The listing builds one solid part. Answer for the finished solid, in the listing's coordinates (mm). A direction names the side the tool comes from. Round coordinates to 2 decimals unless told otherwise and drop trailing zeros. Write each loop counter-clockwise with the first axis right and the second up, starting at its lowest first coordinate (ties: lowest second). Pieces come first, ordered by that corner, then holes. Notation, with made-up numbers: (-36.75, 71) - (-4.75, 71) arc R20 cw to (-4.75, 101) - close; hole circle Ø2 at (-13.75, 50.5). An arc over 180 degrees is marked (long way). Answer in a Markdown table with one row per item.
from build123d import *

# Parameters (mm, degrees)
F0_W     = 58
F0_H     = 63
F1_DEPTH = 29.5
F2_R     = 5
F3_R     = 4
F3_R_2   = 2.5
F4_DEPTH = 4


with BuildPart() as f1:
    # F0 (on Front) → F1 (new body)
    with BuildSketch(Plane.XZ):
        Rectangle(F0_W, F0_H)
    extrude(amount=F1_DEPTH)

    # F2
    f2_edges = [f1.edges().sort_by_distance(p)[0] for p in [
        (0, 0, 31.5),
        (0, 0, -31.5),
        (0, -29.5, -31.5),
        (0, -29.5, 31.5),
    ]]
    fillet(f2_edges, radius=F2_R)

    # F3 (on face) → F4 (join)
    with BuildSketch(Plane.YZ.offset(29)):
        with Locations((-8, 22.752069)):
            Circle(F3_R)
        with Locations((-8, 10.752069)):
            Circle(F3_R_2)
    extrude(amount=F4_DEPTH)


solid = f1.part
(1) Section A-A (y = -8) is taken. Give the vertices of the cut face in (x, z), and give its area (3 significant figures).
Checked values:
| item | result |
|---|---|
| outline | (-29, -31.5) - (29, -31.5) - (29, 8.25) - (33, 8.25) - (33, 13.25) - (29, 13.25) - (29, 18.75) - (33, 18.75) - (33, 26.75) - (29, 26.75) - (29, 31.5) - (-29, 31.5) - close |
| area | 3,710 mm2 |
(2) For faces 5 (the flat face through (0, -15, 31.5)), 6 (the cylindrical face through (30.97, -8.54, 8.31)), determine the directions among +Z, -Z, +X, -X, +Y, -Y from which every point of the face is accessible in a straight line to the end or side of a thin tool.
Checked values:
| item | result |
|---|---|
| face 5 | +Z, +X, -X, +Y, -Y |
| face 6 | +X |
(3) A flat-ended cylindrical pin translates along its axis: pin 1 (3 mm diameter, centred on y = -9, z = -0.5, fed in from +X). Find the tip coordinate at first contact, or state that the pin passes through.
Checked values:
| item | result |
|---|---|
| pin 1 | stops at x = 29 |
(4) For a pull along Z with two mould halves and no side action, classify faces 1 (the flat face through (33, -8, 11)), 2 (the cylindrical face through (0.41, -1.5, -30.07)), 3 (the cylindrical face through (0.41, -28, 30.07)), 4 (the cylindrical face through (30.972, -11.174, 20.318)) as pulls with the +Z half, pulls with the -Z half, needs draft (parallel to the pull), parting line crosses it, or undercut.
Checked values:
| item | result |
|---|---|
| face 1 | needs draft |
| face 2 | pulls with the -Z half |
| face 3 | pulls with the +Z half |
| face 4 | undercut |
(5) Section C-C (y = -17.5) is taken. Give the vertices of the cut face in (x, z).
Checked values:
| item | result |
|---|---|
| outline | (-29, -31.5) - (29, -31.5) - (29, 31.5) - (-29, 31.5) - close |
(6) Find the intervals of material crossed by line 1 (X direction, y = -16.25, z = -14.5); line 2 (Z direction, x = -22.5, y = -25.75); line 3 (Z direction, x = 5, y = -25.25), in increasing order.
Checked values:
| item | result |
|---|---|
| line 1 | x = -29 to 29 |
| line 2 | z = -31.34 to 31.34 |
| line 3 | z = -31.44 to 31.44 |
(7) Section B-B (z = 11.5) is taken. Give the vertices of the cut face in (x, y), and give its area (3 significant figures).
Checked values:
| item | result |
|---|---|
| outline | (-29, -29.5) - (29, -29.5) - (29, -10.39) - (33, -10.39) - (33, -5.61) - (29, -5.61) - (29, 0) - (-29, 0) - close |
| area | 1,730 mm2 |
